Build history of the part. All positions in model axes, mm. Round coordinates to 2 decimals unless told otherwise and drop trailing zeros. Write each loop counter-clockwise with the first axis right and the second up, starting at its lowest first coordinate (ties: lowest second). Pieces come first, ordered by that corner, then holes.
from build123d import *

# Parameters (mm, degrees)
SKETCH1_W           = 236
SKETCH1_H           = 12
BOSS_EXTRUDE1_DEPTH = 6
SKETCH2_R           = 4.8
CUT_EXTRUDE1_DEPTH  = 12


with BuildPart() as part:
    # Sketch1 → Boss-Extrude1 (new, symmetric)
    with BuildSketch(Plane.XY):
        with Locations((60, 0)):
            Rectangle(SKETCH1_W, SKETCH1_H)
    extrude(amount=BOSS_EXTRUDE1_DEPTH, both=True)

    # Sketch2 → Cut-Extrude1 (cut, symmetric)
    with BuildSketch(Plane.XY):
        Circle(SKETCH2_R)
    extrude(amount=CUT_EXTRUDE1_DEPTH, both=True, mode=Mode.SUBTRACT)


solid = part.part
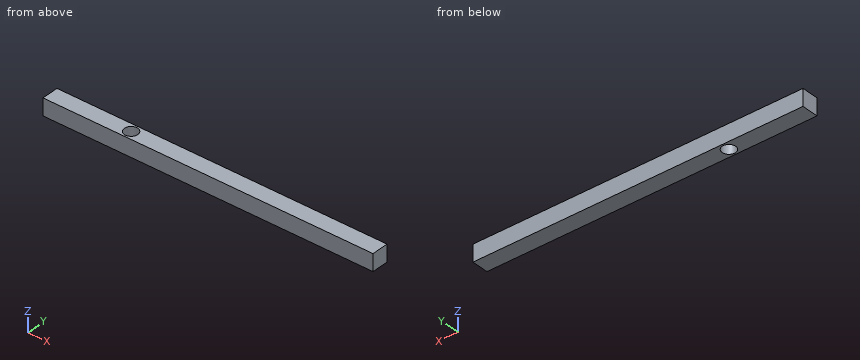
1) Slice it at B-B (x = 0). Write the cut outline in (y, z), plus the area to 3 significant figures.
Results:
outline: (-6, -6) - (-4.8, -6) - (-4.8, 6) - (-6, 6) - close; (4.8, -6) - (6, -6) - (6, 6) - (4.8, 6) - close
area: 28.8 mm2
2) Wall check: L1, parallel to Y at x = 0, z = -1.5; L2, parallel to X at y = -0.5, z = 3; L3, parallel to X at y = -4, z = -0.5. Give the ranges that are in metal, low to high.
Results:
L1: y = -6 to -4.8, 4.8 to 6
L2: x = -58 to -4.77, 4.77 to 178
L3: x = -58 to -2.65, 2.65 to 178
3) Slice it at A-A (y = 0). Write the cut outline in (x, z).
Results:
outline: (-58, -6) - (-4.8, -6) - (-4.8, 6) - (-58, 6) - close; (4.8, -6) - (178, -6) - (178, 6) - (4.8, 6) - close
4) Slice it at C-C (z = -2). Write the cut outline in (x, y).
Results:
outline: (-58, -6) - (178, -6) - (178, 6) - (-58, 6) - close; hole circle Ø9.6 at (0, 0)
